Source: CAD feature listing. Evaluate the final solid. Frame: model axes, mm. Round coordinates to 2 decimals unless told otherwise and drop trailing zeros. Order: outer loops, then holes, each group sorted by start corner. A loop starts at its lowest first (then second) coordinate and runs counter-clockwise, first axis right, second up. Notation, with made-up numbers: (-35, 49.25) -> (-13, 49.25) arc R23 ccw to (-13, 79.25) -> close; hole circle Ø9 at (-22, 59). An arc over 180 degrees is marked (long way). One line per item, written item: value. Start each with the question number.
1) Section B-B (y = 21). Return the cut outline in (x, z), and give its area (3 significant figures).
2) Ray query, L1, parallel to Y at x = 14.5, z = 2.3; L2, parallel to X at y = 7.5, z = 4.6; L3, parallel to X at y = 21.5, z = 2.75. Return the intervals inside material, ascending.
3) Section C-C (z = 4.45). Return the cut outline in (x, y), and give its area (3 significant figures).
4) Pin query (flat end, axial travel): P1, Ø1, axis at x = 31.5, y = 13.5, coming from the -Z side. Return the tip coordinate at first contact, or that it passes through.
5) Section A-A (x = 16). Return the cut outline in (y, z), and give its area (3 significant figures).
6) Mould query, pull axis Y, two halves, no side actions, for faces 1 (the face through (10, 14, 2)), 2 (the face through (39.517, 20.76, 2.465)), 3 (the face through (28, 3, 2)). Classes: pulls with the +Y half, pulls with the -Y half, needs draft (parallel to the pull), parting line crosses it, or undercut.
Autodesk Fusion 360 part; units mm, degrees
sketch "Sketch1" plane through (0, 0, 0) normal (0, 0, 1) x (1, 0, 0)
  line L0 (10, 25) -> (46, 25)
  line L1 (46, 25) -> (46, 3)
  line L2 (46, 3) -> (10, 3)
  line L3 (10, 3) -> (10, 25)
  dimension "d1" = 36
  dimension "d2" = 22
extrude "Extrude1" add sketch "Sketch1" along normal blind 5
sketch "Sketch2" plane through (0, 0, 5) normal (0, 0, 1) x (-1, 0, 0)
  line L0 (-10, -3) -> (-46, -3)
  line L1 (-46, -3) -> (-46, -25)
  line L2 (-46, -25) -> (-10, -25)
  line L3 (-10, -25) -> (-10, -3)
  line L4 (-21.9549, -14.5099) -> (-33.9998, -14.5099)
  line L5 (-33.9998, -14.5099) -> (-33.9998, -13.5007)
  line L6 (-33.9998, -13.5007) -> (-21.9549, -13.5007)
  line L7 (-21.9549, -13.5007) -> (-21.9549, -14.5099)
hole "Hole3" at (14.5003, 20.5001, 5) direction (0, 0, -1) diameter 4 depth 5 tip angle 180
pattern_linear "R-Pattern2" count 2 spacing 13 along (0, -1, 0) count 2 spacing 27 along (1, 0, 0) of "Hole3"

Autodesk Fusion 360 part; units mm, degrees
sketch "Sketch1" plane through (0, 0, 0) normal (0, 0, 1) x (1, 0, 0)
  line L0 (10, 25) -> (46, 25)
  line L1 (46, 25) -> (46, 3)
  line L2 (46, 3) -> (10, 3)
  line L3 (10, 3) -> (10, 25)
  dimension "d1" = 36
  dimension "d2" = 22
extrude "Extrude1" add sketch "Sketch1" along normal blind 0.05
sketch "Sketch5" plane through (0, 0, 0.05) normal (0, 0, 1) x (-1, 0, 0)
  line L0 (-10, -3) -> (-46, -3)
  line L1 (-46, -3) -> (-46, -25)
  line L2 (-46, -25) -> (-10, -25)
  line L3 (-10, -25) -> (-10, -3)
  line L4 (-16.7182, -15.0406) -> (-21.9549, -13.5007)
  line L5 (-21.9549, -14.5099) -> (-16.0325, -16.2515)
  line L6 (-16.7182, -15.0406) -> (-16.0325, -16.2515)
hole "Hole3" at (14.5003, 20.5001, 0.05) direction (0, 0, -1) diameter 4 depth 4 tip angle 180
pattern_linear "R-Pattern2" count 2 spacing 13 along (0, -1, 0) count 2 spacing 27 along (1, 0, 0) of "Hole3"
sketch "Sketch11" plane through (0, 0, 0.05) normal (0, 0, 1) x (-1, 0, 0)
  circle A0 centre (-41.5003, -7.5001) radius 2
  circle A1 centre (-41.5003, -20.5001) radius 2
  circle A2 centre (-14.5003, -7.5001) radius 2
  circle A3 centre (-14.5003, -20.5001) radius 2
  line L0 (-10, -3) -> (-46, -3)
  line L1 (-46, -3) -> (-46, -25)
  line L2 (-46, -25) -> (-10, -25)
  line L3 (-10, -25) -> (-10, -3)
  line L4 (-16.3501, -14.6002) -> (-17.1489, -14.6002)
  line L5 (-17.1489, -14.6002) -> (-17.1489, -14.1)
  line L6 (-17.1489, -14.1) -> (-16.3501, -14.1)
  line L7 (-16.3501, -14.1) -> (-16.3501, -14.6002)
  line L8 (-16.3495, -13.4) -> (-17.1505, -13.4)
  line L9 (-17.1505, -13.4) -> (-17.1505, -13.9)
  line L10 (-17.1505, -13.9) -> (-16.3495, -13.9)
  line L11 (-16.3495, -13.9) -> (-16.3495, -13.4)
extrude "Extrude8" cut sketch "Sketch11" against normal blind 1.6 contours L4 L5 L6 L7 | L8 L9 L10 L11
sketch "Sketch15" plane through (0, 0, 0.05) normal (0, 0, 1) x (-1, 0, 0)
  line L0 (-16.3495, -13.4) -> (-16.3495, -13.9)
  line L1 (-16.3495, -13.9) -> (-17.1505, -13.9)
  line L2 (-17.1505, -13.9) -> (-17.1505, -13.4)
  line L3 (-17.1505, -13.4) -> (-16.3495, -13.4)
  line L4 (-16.3501, -14.6002) -> (-17.1489, -14.6002)
  line L5 (-17.1489, -14.6002) -> (-17.1489, -14.1)
  line L6 (-17.1489, -14.1) -> (-16.3501, -14.1)
  line L7 (-16.3501, -14.1) -> (-16.3501, -14.6002)
  circle A0 centre (-41.5003, -7.5001) radius 2
  circle A1 centre (-41.5003, -20.5001) radius 2
  circle A2 centre (-14.5003, -7.5001) radius 2
  circle A3 centre (-14.5003, -20.5001) radius 2
  line L8 (-10, -3) -> (-46, -3)
  line L9 (-46, -3) -> (-46, -25)
  line L10 (-46, -25) -> (-10, -25)
  line L11 (-10, -25) -> (-10, -3)
  line L12 (-38.8493, -14.6007) -> (-39.6492, -14.6007)
  line L13 (-39.6492, -14.6007) -> (-39.6492, -14.1)
  line L14 (-39.6492, -14.1) -> (-38.8493, -14.1)
  line L15 (-38.8493, -14.1) -> (-38.8493, -14.6007)
  line L16 (-38.8501, -13.9) -> (-39.65, -13.9)
  line L17 (-39.65, -13.9) -> (-39.65, -13.3997)
  line L18 (-39.65, -13.3997) -> (-38.8501, -13.3997)
  line L19 (-38.8501, -13.3997) -> (-38.8501, -13.9)
extrude "Extrude10" cut sketch "Sketch15" against normal blind 1.6 contours L12 L13 L14 L15 | L16 L17 L18 L19
Findings:
1. outline: (10, 0) -> (12.56, 0) -> (12.56, 5) -> (10, 5) -> close; (16.44, 0) -> (39.56, 0) -> (39.56, 5) -> (16.44, 5) -> close; (43.44, 0) -> (46, 0) -> (46, 5) -> (43.44, 5) -> close
1. area: 141 mm2
2. L1: 3 to 5.5, 9.5 to 18.5, 22.5 to 25
2. L2: 10 to 12.5, 16.5 to 39.5, 43.5 to 46
2. L3: 10 to 12.77, 16.23 to 39.77, 43.23 to 46
3. outline: (10, 3) -> (46, 3) -> (46, 25) -> (10, 25) -> close; hole circle Ø4 at (14.5, 7.5); hole circle Ø4 at (14.5, 20.5); hole circle Ø4 at (41.5, 7.5); hole circle Ø4 at (41.5, 20.5)
3. area: 742 mm2
4. P1: z = 0
5. outline: (3, 0) -> (6.18, 0) -> (6.18, 5) -> (3, 5) -> close; (8.82, 0) -> (19.18, 0) -> (19.18, 5) -> (8.82, 5) -> close; (21.82, 0) -> (25, 0) -> (25, 5) -> (21.82, 5) -> close
5. area: 83.5 mm2
6. face 1: needs draft
6. face 2: undercut
6. face 3: pulls with the -Y half
